Part model, mm, in its own coordinate system. A direction names the side the tool comes from. Round coordinates to 2 decimals unless told otherwise and drop trailing zeros. Loops run counter-clockwise (first coordinate to the right, second up) from the corner with the lowest first, then second, coordinate; pieces in that order, holes last. Notation, with made-up numbers: (-8, 83.25) -> (14, 83.25) arc R18 ccw to (14, 100.25) -> close; hole circle Ø9 at (-4.75, -10). An arc over 180 degrees is marked (long way). Answer as CSV lines item,"result".
Autodesk Fusion 360 part; units mm, degrees
sketch "Sketch1" plane through (0, 0, 0) normal (0, 1, 0) x (1, 0, 0)
  line L0 (-67, -114.8999) -> (-57, -114.8999)
  line L1 (-57, -114.8999) -> (-57, -54.8999)
  line L2 (-57, -54.8999) -> (57, -54.8999)
  line L3 (57, -54.8999) -> (57, -114.8999)
  line L4 (57, -114.8999) -> (67, -114.8999)
  line L5 (67, -114.8999) -> (67, -44.8999)
  line L6 (67, -44.8999) -> (-67, -44.8999)
  line L7 (-67, -44.8999) -> (-67, -114.8999)
  dimension "d2" = 67
  dimension "d3" = 10
  dimension "d6" = 70
  dimension "d16" = 10
  dimension "d17" = 10
  dimension "d31" = 67
extrude "Extrude1" add sketch "Sketch1" along normal blind 35
sketch "Sketch3" plane through (-67, 0, 0) normal (-1, 0, 0) x (0, -1, 0)
  line L0 (0, 44.8999) -> (0, 114.8999)
  line L1 (0, 114.8999) -> (-35, 114.8999)
  line L2 (-35, 114.8999) -> (-35, 44.8999)
  line L3 (-35, 44.8999) -> (0, 44.8999)
  circle A0 centre (-17.5, 99.8999) radius 1
  dimension "d12" = 2
  dimension "d15" = 17.5
  dimension "d24" = 15
extrude "Extrude2" cut sketch "Sketch3" against normal blind 101 contours A0
sketch "Sketch4" plane through (0, 35, 0) normal (0, 1, 0) x (-1, 0, 0)
  line L0 (67, 44.8999) -> (67, 114.8999)
  line L1 (67, 114.8999) -> (57, 114.8999)
  line L2 (57, 114.8999) -> (57, 54.8999)
  line L3 (57, 54.8999) -> (-57, 54.8999)
  line L4 (-57, 54.8999) -> (-57, 114.8999)
  line L5 (-57, 114.8999) -> (-67, 114.8999)
  line L6 (-67, 114.8999) -> (-67, 44.8999)
  line L7 (-67, 44.8999) -> (67, 44.8999)
  line L8 (-5, 52.3999) -> (1, 52.3999)
  line L9 (1, 52.3999) -> (1, 47.3999)
  line L10 (1, 47.3999) -> (-5, 47.3999)
  line L11 (-5, 47.3999) -> (-5, 52.3999)
  line L12 (-5, 52.3999) -> (1, 47.3999) construction
  line L13 (1, 52.3999) -> (-5, 47.3999) construction
  point P0 (-2, 49.8999)
  dimension "d18" = 5
  dimension "d19" = 6
  dimension "d20" = 5
  dimension "d21" = 65
extrude "Extrude3" cut sketch "Sketch4" against normal blind 20 contours L8 L9 L10 L11
mirror "Mirror2" about plane through (0, 0, 0) normal (1, 0, 0) of "Extrude2"
fillet "Fillet2" radius 0.5 2 edges at (67, 18.4323, 99.5383) (-67, 18.4323, 100.2615)
Q1. Two-plate mould, pull along X, no slides. Class faces 1 (the face through (-67, 17, 79)), 2 (the face through (5, 25, 50)), 3 (the face through (2, 15, 50)), 4 (the face through (62, 17, 114.9)): pulls with the +X half, pulls with the -X half, needs draft (parallel to the pull), parting line crosses it, or undercut.
Geometry results:
face 1,"pulls with the -X half"
face 2,"undercut"
face 3,"undercut"
face 4,"needs draft"
Q2. Which spindle directions (+Z, -Z, +X, -X, +Y, -Y) get a long thin tool onto all of the face, cutting with end or side? Do faces 5 (the face through (-57, 17, 85)), 6 (the face through (-62, 17, 114.9)), 7 (the face through (2, 25, 52.4)). Say none if no direction does.
Geometry results:
face 5,"+Z, +Y, -Y"
face 6,"+Z, +X, -X, +Y, -Y"
face 7,"+Y"
Q3. Saw through at A-A, the plane z = 86. Write the cut outline in (x, y).
Geometry results:
outline,"(-67, 0) -> (-57, 0) -> (-57, 35) -> (-67, 35) -> close; (57, 0) -> (67, 0) -> (67, 35) -> (57, 35) -> close"
Q4. Drop flat-ended pins along their axis: P1, Ø10.5, axis at x = -22, y = 14.5, coming from the +Z side; P2, Ø2.5, axis at y = 17.5, z = 99.9, coming from the -X side; P3, Ø1.5, axis at x = 2, z = 51, coming from the +Y side; P4, Ø8, axis at x = -19.5, z = 56.5, coming from the -Y side. Give the stop position or say it passes through.
Geometry results:
P1,"z = 54.9"
P2,"x = -66.93"
P3,"y = 15"
P4,"y = 0"
Q5. Drill centre lines: line 1 along X through (y, z) = (10, 108.5); line 2 along Z through (x, y) = (59.5, 17.5); line 3 along Z through (x, y) = (-45.5, 7). Where is each one in solid material? Low to high.
Geometry results:
line 1,"-67 to -57, 57 to 67"
line 2,"44.9 to 98.9, 100.9 to 114.9"
line 3,"44.9 to 54.9"
Q6. Saw through at C-C, the plane x = 1. Write the cut outline in (y, z).
Geometry results:
outline,"(0, 44.9) -> (35, 44.9) -> (35, 47.4) -> (15, 47.4) -> (15, 52.4) -> (35, 52.4) -> (35, 54.9) -> (0, 54.9) -> close"
Q7. Saw through at B-B, the plane y = 26. Write the cut outline in (x, z), then the cut area to 3 significant figures.
Geometry results:
outline,"(-67, 44.9) -> (67, 44.9) -> (67, 114.9) -> (57, 114.9) -> (57, 54.9) -> (-57, 54.9) -> (-57, 114.9) -> (-67, 114.9) -> close; hole (-1, 47.4) -> (5, 47.4) -> (5, 52.4) -> (-1, 52.4) -> close"
area,"2,510 mm2"
Q8. Saw through at D-D, the plane y = 12. Write the cut outline in (x, z).
Geometry results:
outline,"(-67, 44.9) -> (67, 44.9) -> (67, 114.9) -> (57, 114.9) -> (57, 54.9) -> (-57, 54.9) -> (-57, 114.9) -> (-67, 114.9) -> close"
